Autodesk Inventor part; units mm, degrees
ref_plane "YZ Plane" through (0, 0, 0) normal (1, 0, 0) x (0, 1, 0)
ref_plane "XZ Plane" through (0, 0, 0) normal (0, 1, 0) x (-1, 0, 0)
ref_plane "XY Plane" through (0, 0, 0) normal (0, 0, 1) x (1, 0, 0)
sketch "Sketch1" plane through (0, 0, 0) normal (0, 1, 0) x (-1, 0, 0)
  line L0 (-101.0152, -60.2536) -> (98.9848, -60.2536)
  line L1 (98.9848, -60.2536) -> (98.9848, 149.7464)
  line L2 (98.9848, 149.7464) -> (-101.0152, 149.7464)
  line L3 (-101.0152, 149.7464) -> (-101.0152, -60.2536)
  line L4 (-101.0152, -60.2536) -> (98.9848, 149.7464) construction
  line L5 (98.9848, -60.2536) -> (-101.0152, 149.7464) construction
  line L6 (-65.0152, -60.2536) -> (62.9848, -60.2536)
  line L7 (62.9848, -60.2536) -> (62.9848, -45.2536)
  line L8 (62.9848, -45.2536) -> (-65.0152, -45.2536)
  line L9 (-65.0152, -45.2536) -> (-65.0152, -60.2536)
  line L10 (98.9848, -35.2536) -> (76.9848, -35.2536)
  line L11 (76.9848, -35.2536) -> (76.9848, 34.7464)
  line L12 (76.9848, 34.7464) -> (98.9848, 34.7464)
  line L13 (98.9848, 34.7464) -> (98.9848, -35.2536)
  line L14 (-101.0152, -35.2536) -> (-79.0152, -35.2536)
  line L15 (-79.0152, -35.2536) -> (-79.0152, 34.7464)
  line L16 (-79.0152, 34.7464) -> (-101.0152, 34.7464)
  line L17 (-101.0152, 34.7464) -> (-101.0152, -35.2536)
  line L18 (84.9848, 37.2464) -> (94.9848, 37.2464)
  line L19 (94.9848, 37.2464) -> (94.9848, 42.2464)
  line L20 (94.9848, 42.2464) -> (84.9848, 42.2464)
  line L21 (84.9848, 42.2464) -> (84.9848, 37.2464)
  line L22 (84.9848, 37.2464) -> (94.9848, 42.2464) construction
  line L23 (94.9848, 37.2464) -> (84.9848, 42.2464) construction
  line L24 (-97.0152, 37.2464) -> (-87.0152, 37.2464)
  line L25 (-87.0152, 37.2464) -> (-87.0152, 42.2464)
  line L26 (-87.0152, 42.2464) -> (-97.0152, 42.2464)
  line L27 (-97.0152, 42.2464) -> (-97.0152, 37.2464)
  line L28 (-97.0152, 37.2464) -> (-87.0152, 42.2464) construction
  line L29 (-87.0152, 37.2464) -> (-97.0152, 42.2464) construction
  line L30 (-78.5152, 2.7464) -> (-72.5152, 2.7464)
  line L31 (-72.5152, 2.7464) -> (-72.5152, -8.2536)
  line L32 (-72.5152, -8.2536) -> (-78.5152, -8.2536)
  line L33 (-78.5152, -8.2536) -> (-78.5152, 2.7464)
  line L34 (70.4848, 2.7464) -> (76.4848, 2.7464)
  line L35 (76.4848, 2.7464) -> (76.4848, -8.2536)
  line L36 (76.4848, -8.2536) -> (70.4848, -8.2536)
  line L37 (70.4848, -8.2536) -> (70.4848, 2.7464)
  line L38 (-101.0152, 149.7464) -> (-97.0152, 149.7464)
  circle A0 centre (-99.0152, 147.6464) radius 1
  line L39 (-101.0152, -60.2536) -> (-97.0152, -60.2536)
  line L40 (-101.0152, -36.2536) -> (-101.0152, -60.2536)
  circle A1 centre (-99.0152, -58.1536) radius 1
  circle A2 centre (-99.0152, -38.2536) radius 1
  circle A3 centre (-99.0152, 97.6464) radius 1
  circle A4 centre (-99.0152, 52.6464) radius 1
  circle A5 centre (-69.0152, -58.1536) radius 1
  circle A6 centre (96.9848, -58.1536) radius 1
  circle A7 centre (66.9848, -58.1536) radius 1
  circle A8 centre (96.9848, -38.2536) radius 1
  circle A9 centre (96.9848, 52.6464) radius 1
  circle A10 centre (96.9848, 97.6464) radius 1
  circle A11 centre (96.9848, 147.6464) radius 1
  circle A12 centre (66.9848, 147.6464) radius 1
  circle A13 centre (-69.0152, 147.6464) radius 1.0002
  circle A14 centre (-1.0152, 147.6464) radius 1
  point P0 (-1.0152, 44.7464)
  point P1 (89.9848, 39.7464)
  point P2 (-92.0152, 39.7464)
  point P3 (-101.0152, 34.7464)
  point P4 (98.9848, 34.7464)
  point P5 (62.9848, -60.2536)
  point P6 (-90.0152, -35.2536)
  point P7 (87.9848, 34.7464)
  point P8 (-90.0152, 34.7464)
  point P9 (-99.0152, -60.2536)
  point P10 (-99.0152, 149.7464)
  dimension "d22" = 200
  dimension "d23" = 210
  dimension "d24" = 15
  dimension "d25" = 128
  dimension "d26" = 36
  dimension "d27" = 22
  dimension "d28" = 70
  dimension "d29" = 10
  dimension "d30" = 22
  dimension "d31" = 70
  dimension "d32" = 10
  dimension "d33" = 5
  dimension "d34" = 10
  dimension "d35" = 5
  dimension "d58" = 10
  dimension "d70" = 5
  dimension "d71" = 11
  dimension "d72" = 6
  dimension "d73" = 52
  dimension "d74" = 22.5
  dimension "d75" = 6
  dimension "d76" = 11
  dimension "d77" = 52
  dimension "d78" = 22.5
  dimension "d83" = 4
  dimension "d84" = 4
  dimension "d85" = 5
  dimension "d88" = 2
  dimension "d91" = 2
  dimension "d92" = 2
  dimension "d93" = 22
  dimension "d94" = 2.1
  dimension "d95" = 2
  dimension "d96" = 2
  dimension "d97" = 2.1
  dimension "d98" = 2
  dimension "d99" = 50
  dimension "d100" = 2
  dimension "d101" = 95
  dimension "d102" = 2
  dimension "d104" = 2
  dimension "d105" = 2
  dimension "d106" = 2.1
  dimension "d107" = 2.1
  dimension "d108" = 2
  dimension "d109" = 22
  dimension "d112" = 2.1
  dimension "d113" = 32
  dimension "d114" = 2.1
  dimension "d115" = 32
  dimension "d116" = 32
  dimension "d117" = 2.1
  dimension "d118" = 2
  dimension "d119" = 2.1
  dimension "d120" = 100
  dimension "d122" = 2
  dimension "d123" = 2
  dimension "d124" = 2
  dimension "d125" = 2
  dimension "d126" = 2
  dimension "d178" = 32
  dimension "d179" = 50
  dimension "d180" = 95
extrude "Body" add sketch "Sketch1" along normal blind 3 contours L3 L14 L15 L16 L2 L1 L12 L11 L10 L0 L7 L8 L9
sketch "Sketch3" plane through (0, 3, 0) normal (0, 1, 0) x (1, 0, 0)
  line L0 (65.0152, 60.2536) -> (65.0152, 45.2536)
  line L1 (-62.9848, 60.2536) -> (-98.9848, 60.2536)
  line L2 (65.0152, 45.2536) -> (-62.9848, 45.2536)
  line L3 (-62.9848, 45.2536) -> (-62.9848, 60.2536)
  line L4 (-62.9848, 60.2536) -> (65.0152, 60.2536)
  line L5 (65.0152, 60.2536) -> (65.0152, 45.2536)
  circle A0 centre (60.0152, 48.2536) radius 2
  circle A1 centre (60.0152, 57.2536) radius 2
  circle A2 centre (38.0152, 48.2536) radius 2
  circle A3 centre (-57.9848, 57.2536) radius 2
  circle A4 centre (-57.9848, 48.2536) radius 2
  circle A5 centre (-35.9848, 48.2536) radius 2
  point P0 (0, 0)
  point P1 (65.0152, 60.2536)
  dimension "d38" = 4
  dimension "d39" = 5
  dimension "d40" = 3
  dimension "d41" = 4
  dimension "d42" = 3
  dimension "d43" = 5
  dimension "d44" = 4
  dimension "d45" = 27
  dimension "d46" = 3
  dimension "d47" = 4
  dimension "d48" = 3
  dimension "d49" = 5
  dimension "d50" = 4
  dimension "d51" = 5
  dimension "d52" = 3
  dimension "d53" = 4
  dimension "d54" = 3
  dimension "d55" = 27
extrude "IRSensor" add sketch "Sketch3" against normal blind 3
sketch "Sketch4" plane through (0, 3, 0) normal (0, 1, 0) x (1, 0, 0)
  line L0 (101.0152, -34.7464) -> (79.0152, -34.7464)
  line L1 (79.0152, -34.7464) -> (79.0152, 35.2536)
  line L2 (79.0152, 35.2536) -> (101.0152, 35.2536)
  line L3 (101.0152, 35.2536) -> (101.0152, -34.7464)
  point P0 (0, 0)
extrude "RodaKrMark" add sketch "Sketch4" against normal blind 3
sketch "Sketch5" plane through (0, 3, 0) normal (0, 1, 0) x (1, 0, 0)
  line L0 (-76.9848, 35.2536) -> (-76.9848, -34.7464)
  line L1 (-98.9848, 35.2536) -> (-76.9848, 35.2536)
  line L2 (-76.9848, -34.7464) -> (-98.9848, -34.7464)
  line L3 (-98.9848, -34.7464) -> (-98.9848, 35.2536)
  line L4 (-98.9848, 35.2536) -> (-76.9848, 35.2536)
  line L5 (-76.9848, 35.2536) -> (-76.9848, -34.7464)
  point P0 (0, 0)
extrude "RodaKaMark" add sketch "Sketch5" against normal blind 3
sketch "Sketch6" plane through (0, 3, 0) normal (0, 1, 0) x (1, 0, 0)
  line L0 (78.5152, -2.7464) -> (72.5152, -2.7464)
  line L1 (72.5152, 8.2536) -> (78.5152, 8.2536)
  line L2 (78.5152, -2.7464) -> (72.5152, -2.7464)
  line L3 (72.5152, -2.7464) -> (72.5152, 8.2536)
  line L4 (72.5152, 8.2536) -> (78.5152, 8.2536)
  line L5 (78.5152, 8.2536) -> (78.5152, -2.7464)
  point P0 (0, 0)
extrude "Extrusion5" add sketch "Sketch6" against normal blind 25
sketch "Sketch8" plane through (0, 3, 0) normal (0, 1, 0) x (1, 0, 0)
  line L0 (-76.4848, -2.7464) -> (-76.4848, 8.2536)
  line L1 (-76.4848, 8.2536) -> (-70.4848, 8.2536)
  line L2 (-70.4848, 8.2536) -> (-70.4848, -2.7464)
  line L3 (-70.4848, -2.7464) -> (-76.4848, -2.7464)
  line L4 (-76.4848, -2.7464) -> (-76.4848, 8.2536)
  point P0 (0, 0)
extrude "Extrusion6" add sketch "Sketch8" against normal blind 25
sketch "Sketch9" plane through (78.5152, 0, 2.7464) normal (1, 0, 0) x (0, 0, -1)
  line L0 (11, 0) -> (11, -22)
  line L1 (63, 0) -> (-147, 0)
  line L2 (11, -22) -> (0, -22)
  line L3 (0, -22) -> (0, 0)
  line L4 (0, 0) -> (11, 0)
  line L5 (11, 0) -> (11, -22)
  circle A0 centre (5.5, -4.887) radius 1.5
  circle A1 centre (5.5, -15.887) radius 1.5
  point P0 (2.7464, 0)
  dimension "d146" = 11
  dimension "d147" = 3
  dimension "d148" = 3
  dimension "d149" = 11
hole "BautBawah" at (78.5152, -15.887, -2.7536) direction (-1, 0, 0) diameter 3 end through all
sketch "Sketch10" plane through (78.5152, 0, 2.7464) normal (1, 0, 0) x (0, 0, -1)
  point P0 (2.7464, 0)
  point P1 (5.5237, -4.8856)
hole "Hole2" at (78.5152, -4.8856, -2.7773) direction (-1, 0, 0) diameter 3 end through all
sketch "Sketch11" plane through (78.5152, 0, 2.7464) normal (1, 0, 0) x (0, 0, -1)
  point P0 (2.7464, 0)
  point P1 (5.5357, -4.6342)
hole "Hole3" at (78.5152, -4.6342, -2.7892) direction (-1, 0, 0) diameter 3 end through all
sketch "Sketch12" plane through (78.5152, 0, 2.7464) normal (1, 0, 0) x (0, 0, -1)
  point P0 (2.7464, 0)
  point P1 (5.5238, -4.1202)
hole "Hole4" at (78.5152, -4.1202, -2.7774) direction (-1, 0, 0) diameter 3 end through all
sketch "Sketch13" plane through (78.5152, 0, 2.7464) normal (1, 0, 0) x (0, 0, -1)
  point P0 (2.7464, 0)
  point P1 (5.5033, -3.3695)
hole "Hole5" at (78.5152, -3.3695, -2.7569) direction (-1, 0, 0) diameter 3 end through all
sketch "Sketch14" plane through (78.5152, 0, 2.7464) normal (1, 0, 0) x (0, 0, -1)
  point P0 (2.7464, 0)
  point P1 (5.5284, -2.8201)
hole "Hole6" at (78.5152, -2.8201, -2.782) direction (-1, 0, 0) diameter 3 end through all
properties part number "DesignBawahRobot"
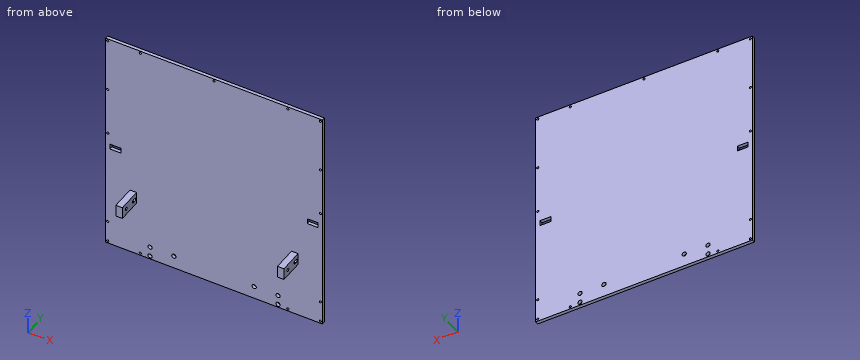
For this review, take the finished solid that the model builds, in its own axes (mm). Round coordinates to 2 decimals unless told otherwise and drop trailing zeros. Loops run counter-clockwise (first coordinate to the right, second up) from the corner with the lowest first, then second, coordinate; pieces in that order, holes last.
Q1. Insertion check: pin 1 Ø3 at (x, z) = (-66.98, -58.15) entering from -Y; pin 2 Ø2.5 at (x, z) = (99.02, 52.65) entering from +Y; pin 3 Ø4 at (y, z) = (-4.89, -2.78) entering from -X; pin 4 Ø6.5 at (x, y) = (-73.5, -10.5) entering from -Z. Each pin has a flat end and moves straight along its axis. Give the tip position at first contact, or say it passes through.
Result sheet:
pin 1: stops at y = 0
pin 2: stops at y = 3
pin 3: stops at x = -76.48
pin 4: stops at z = -8.25
Q2. Add section B-B on z = 24.5. Write out the cut boundary in (x, y).
Result sheet:
outline: (-98.98, 0) - (101.02, 0) - (101.02, 3) - (-98.98, 3) - close
Q3. Add section C-C on x = 8.5. Write out the cut boundary in (y, z).
Result sheet:
outline: (0, -60.25) - (3, -60.25) - (3, 149.75) - (0, 149.75) - close
Q4. Add section A-A on y = -10.5. Write out the cut boundary in (x, z), plus the area to 3 significant figures.
Result sheet:
outline: (-76.48, -8.25) - (-70.48, -8.25) - (-70.48, 2.75) - (-76.48, 2.75) - close; (72.52, -8.25) - (78.52, -8.25) - (78.52, 2.75) - (72.52, 2.75) - close
area: 132 mm2
Q5. To check wall thickness, follow line 1 along X through (y, z) = (-13, -2.5); line 2 along Y through (x, z) = (-17, 48); line 3 along Z through (x, y) = (-73, -1.75). State the ranges of each line that lie inside material, in increasing order.
Result sheet:
line 1: x = -76.48 to -70.48, 72.52 to 78.52
line 2: y = 0 to 3
line 3: z = -8.25 to -3.83, -1.73 to 2.75
